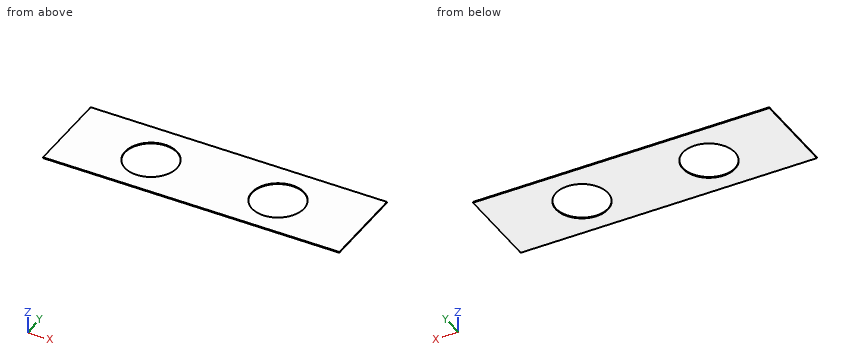
from build123d import *

# Parameters (mm, degrees)
SKETCH1_W           = 1066.8
SKETCH1_H           = 311.15
BOSS_EXTRUDE1_DEPTH = 3.175
CUT_EXTRUDE1_REACH  = 5.175
SKETCH2_R           = 93.6625


with BuildPart() as part:
    # Sketch1 → Boss-Extrude1 (new body)
    with BuildSketch(Plane.XY):
        Rectangle(SKETCH1_W, SKETCH1_H)
    extrude(amount=BOSS_EXTRUDE1_DEPTH)

    # Sketch2 → Cut-Extrude1 (cut, up to next)
    with BuildSketch(Plane.XY.offset(3.175), mode=Mode.PRIVATE) as cut_extrude1_sk1:
        with Locations((228.6, -3.175)):
            Circle(SKETCH2_R)
    cut_extrude1_tool1 = extrude(cut_extrude1_sk1.sketch, amount=-CUT_EXTRUDE1_REACH, mode=Mode.PRIVATE) & part.part
    add(cut_extrude1_tool1.solids().sort_by_distance((228.6, -3.175, 3.175))[0], mode=Mode.SUBTRACT)
    # Sketch2 → Cut-Extrude1 (cut, up to next)
    with BuildSketch(Plane.XY.offset(3.175), mode=Mode.PRIVATE) as cut_extrude1_sk2:
        with Locations((-228.6, -3.175)):
            Circle(SKETCH2_R)
    cut_extrude1_tool2 = extrude(cut_extrude1_sk2.sketch, amount=-CUT_EXTRUDE1_REACH, mode=Mode.PRIVATE) & part.part
    add(cut_extrude1_tool2.solids().sort_by_distance((-228.6, -3.175, 3.175))[0], mode=Mode.SUBTRACT)


solid = part.part
Model file for the job. Use its own axes, mm. Coordinates: 2 decimals unless noted, no trailing zeros. Loops run counter-clockwise (first coordinate to the right, second up) from the corner with the lowest first, then second, coordinate; pieces in that order, holes last. Notation, with made-up numbers: (85, 12.25) -> (120, 12.25) arc R22 cw to (120, 22.25) -> close; hole circle Ø4 at (1, 80.25). An arc over 180 degrees is marked (long way). Use one line per item in the form item = value. Start each with the question number.
(1) Cut at C-C on z = 1.15. Give the cut face in (x, y) (1 decimal).
(2) Probe probe 1 along X at (y, z) = (63.5, 0.45); probe 2 along Y at (x, z) = (-228.6, 1.55) (1 decimal); probe 3 along X at (y, z) = (-63.5, 2.6). List the from-to ranges inside material, lowest first. Write a range as from..to.
(3) Cut at B-B on y = -21. Give the cut face in (x, z) (3 decimals).
(4) Cut at D-D on x = -236. Give the cut face in (y, z) (3 decimals), and give its area (3 significant figures).
(5) Cut at A-A on x = 228.6. Give the cut face in (y, z) (1 decimal), and give its area (3 significant figures).
Values:
q1.outline = (-533.4, -155.6) -> (533.4, -155.6) -> (533.4, 155.6) -> (-533.4, 155.6) -> close; hole circle Ø187.3 at (-228.6, -3.2); hole circle Ø187.3 at (228.6, -3.2)
q2.probe_1 = -533.4..-294.38, -162.82..162.82, 294.38..533.4
q2.probe_2 = -155.6..-96.8, 90.5..155.6
q2.probe_3 = -533.4..-300.25, -156.95..156.95, 300.25..533.4
q3.outline = (-533.4, 0) -> (-320.551, 0) -> (-320.551, 3.175) -> (-533.4, 3.175) -> close; (-136.649, 0) -> (136.649, 0) -> (136.649, 3.175) -> (-136.649, 3.175) -> close; (320.551, 0) -> (533.4, 0) -> (533.4, 3.175) -> (320.551, 3.175) -> close
q4.outline = (-155.575, 0) -> (-96.545, 0) -> (-96.545, 3.175) -> (-155.575, 3.175) -> close; (90.195, 0) -> (155.575, 0) -> (155.575, 3.175) -> (90.195, 3.175) -> close
q4.area = 395 mm2
q5.outline = (-155.6, 0) -> (-96.8, 0) -> (-96.8, 3.2) -> (-155.6, 3.2) -> close; (90.5, 0) -> (155.6, 0) -> (155.6, 3.2) -> (90.5, 3.2) -> close
q5.area = 393 mm2
